Geometry check sheet. Reference: the model listing, model coordinates, mm. Face numbers are marked on the shaded views. A direction names the side the tool comes from. Coordinates: 2 decimals unless noted, no trailing zeros. Write each loop counter-clockwise with the first axis right and the second up, starting at its lowest first coordinate (ties: lowest second). Pieces come first, ordered by that corner, then holes.
Autodesk Inventor part; units mm, degrees
ref_plane "YZ Plane" through (0, 0, 0) normal (1, 0, 0) x (0, 1, 0)
ref_plane "XZ Plane" through (0, 0, 0) normal (0, 1, 0) x (-1, 0, 0)
ref_plane "XY Plane" through (0, 0, 0) normal (0, 0, 1) x (1, 0, 0)
sketch "Sketch1" plane through (0, 0, 0) normal (0, 0, 1) x (1, 0, 0)
  circle A0 centre (0, 0) radius 12.5
  dimension "d0" = 25
extrude "Extrusion1" add sketch "Sketch1" along normal blind 40
sketch "Sketch2" plane through (0, 0, 40) normal (0, 0, 1) x (1, 0, 0)
  point P0 (0, 0)
sketch "Sketch3" plane through (0, 0, 40) normal (0, 0, 1) x (1, 0, 0)
  line L0 (-2.5708, 11.9347) -> (2.7411, 11.9347)
  line L1 (2.7411, 11.9347) -> (2.7411, 11.3559)
  line L2 (2.7411, 11.3559) -> (-2.5708, 11.3559)
  line L3 (-2.5708, 11.3559) -> (-2.5708, 11.9347)
  point P0 (0, 0)
extrude "Extrusion2" add sketch "Sketch3" along normal blind 5
sketch "Sketch5" plane through (-2.5708, 11.9347, 40) normal (0, 1, 0) x (1, 0, 0)
  circle A0 centre (2.5708, -0.9862) radius 1
  point P0 (2.5708, 40)
  dimension "d9" = 2
extrude "Extrusion4" cut sketch "Sketch5" against normal blind 5
sketch "Sketch6" plane through (0, 0, 0) normal (0, 0, -1) x (-1, 0, 0)
  circle A0 centre (0, 0) radius 3
extrude "Extrusion5" add sketch "Sketch6" along normal blind 25
fillet "Fillet1" radius 1 1 edges at (-12.5, 0, 0)
sketch "Sketch7" plane through (-2.5708, 11.9347, 45) normal (0, 1, 0) x (1, 0, 0)
  point P0 (2.5708, 45)
properties part number "DC MOTOR" material "Iron, Gray"
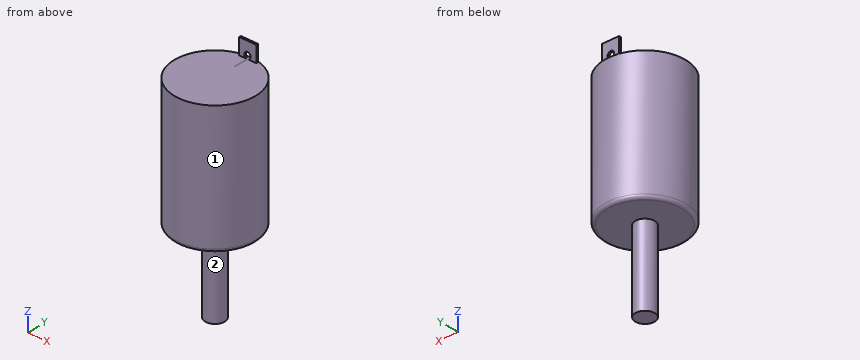
1. Gauge pin test, flat ends, axial feed: pin 1 Ø0.5 at (y, z) = (11.5, 41.5) entering from +X; pin 2 Ø4 at (x, y) = (-5, -6) entering from +Z; pin 3 Ø3 at (x, z) = (0, 40.99) entering from +Y; pin 4 Ø1.5 at (y, z) = (-3, 19.5) entering from -X. Record the tip position at first contact, or that the pin passes through.
Computed values:
pin 1: stops at x = 2.74
pin 2: stops at z = 40
pin 3: stops at y = 12.5
pin 4: stops at x = -12.3
2. Thickness scan on line 1 along Z through (x, y) = (4, -6); line 2 along Z through (x, y) = (9, -8); line 3 along Y through (x, z) = (-2.5, 29.5). Record the ranges inside material, lowest first.
Computed values:
line 1: z = 0 to 40
line 2: z = 0.16 to 40
line 3: y = -12.25 to 12.25
3. Access from +Z, -Z, +X, -X, +Y, -Y to the whole of each face (thin tool, end or side, straight path). Record for the marked faces 1 and 2.
Computed values:
face 1: +Z, -Z
face 2: -Z
4. Sectioned sample at A-A, the plane y = 0. Record the boundary of the cut face in (x, z).
Computed values:
outline: (-12.5, 1) arc R1 ccw to (-11.5, 0) - (-3, 0) - (-3, -25) - (3, -25) - (3, 0) - (11.5, 0) arc R1 ccw to (12.5, 1) - (12.5, 40) - (-12.5, 40) - close
5. Sectioned sample at B-B, the plane z = 12.5. Record the boundary of the cut face in (x, y), and give its area (3 significant figures).
Computed values:
outline: circle Ø25 at (0, 0)
area: 491 mm2
